Here's how the part is built. I have some questions about the finished solid (model axes, mm). Give positions to 0.01 mm unless a question says otherwise; leave off trailing zeros.
Q1. Suppose I cut it at A-A (z = 1.3). Count the separate pieces of the cut face and the enclosed holes in it, and give its area (3 significant figures).
Q2. I need wall thicknesses on probe 1 along Y at (x, z) = (66.04, 1.15) (1 decimal); probe 2 along X at (y, z) = (-14, 1.35); probe 3 along Y at (x, z) = (-20.32, 0.6) (1 decimal). Which ranges of each line are inside material? Lowest first, please.
Q3. I'm going to push flat-ended pins straight in: P1, Ø1.5, axis at x = 37.5, y = 124, coming from the -Z side; P2, Ø0.8, axis at y = -15.5, z = 0.5, coming from the +X side; P3, Ø0.8, axis at x = 59.5, z = 0.5, coming from the +Y side. Where does each tip first touch, or does it pass through?
```python
from build123d import *

# Parameters (mm, degrees)
F0_W     = 1.5875
F0_H     = 10
F0_H_2   = 20
F0_W_2   = 1.74625
F0_H_3   = 5.15
F0_W_3   = 5.15
F0_H_4   = 1.74625
F0_W_4   = 200
F0_H_5   = 1.5875
F0_W_5   = 50
F0_R     = 1.4732
F0_W_6   = 25
F0_H_6   = 30
F0_W_7   = 10
F0_W_8   = 20
F1_DEPTH = 1.5875


# Not quite as in the source:
# - a length typed as a fraction of an inch, garbled in the dataset ("3 / 203.2 mm" for 3/8 in), is restored


with BuildPart() as f1:
    # F0 (on Top) → F1 (new body)
    with BuildSketch(Plane.XY):
        with Locations((-100.79375, 176.5875)):
            Rectangle(F0_W, F0_H)
        with Locations((-100.79375, 36.5875)):
            Rectangle(F0_W, F0_H)
        with Locations((-100.79375, 61.5875)):
            Rectangle(F0_W, F0_H_2)
        with Locations((100.79375, 176.5875)):
            Rectangle(F0_W, F0_H)
        with Locations((100.79375, 36.5875)):
            Rectangle(F0_W, F0_H)
        with Locations((100.79375, 61.5875)):
            Rectangle(F0_W, F0_H_2)
        Polygon((100, 10), (100, 20), (-100, 20), (-100, 10), (-100, -10), (-100, -20), (100, -20), (100, -10), align=None)
        with Locations((-64.2875, -15)):
            Rectangle(F0_W_2, F0_H_3, mode=Mode.SUBTRACT)
        with Locations((-58.414375, -15)):
            Rectangle(F0_W_3, F0_H_4, mode=Mode.SUBTRACT)
        with Locations((-64.2875, 15)):
            Rectangle(F0_W_2, F0_H_3, mode=Mode.SUBTRACT)
        with Locations((-58.414375, 15)):
            Rectangle(F0_W_3, F0_H_4, mode=Mode.SUBTRACT)
        with Locations((-38.414375, -15)):
            Rectangle(F0_W_3, F0_H_4, mode=Mode.SUBTRACT)
        with Locations((-14.2875, -15)):
            Rectangle(F0_W_2, F0_H_3, mode=Mode.SUBTRACT)
        with Locations((-38.414375, 15)):
            Rectangle(F0_W_3, F0_H_4, mode=Mode.SUBTRACT)
        with Locations((-14.2875, 15)):
            Rectangle(F0_W_2, F0_H_3, mode=Mode.SUBTRACT)
        with Locations((14.2875, -15)):
            Rectangle(F0_W_2, F0_H_3, mode=Mode.SUBTRACT)
        with Locations((38.414375, -15)):
            Rectangle(F0_W_3, F0_H_4, mode=Mode.SUBTRACT)
        with Locations((14.2875, 15)):
            Rectangle(F0_W_2, F0_H_3, mode=Mode.SUBTRACT)
        with Locations((38.414375, 15)):
            Rectangle(F0_W_3, F0_H_4, mode=Mode.SUBTRACT)
        with Locations((58.414375, -15)):
            Rectangle(F0_W_3, F0_H_4, mode=Mode.SUBTRACT)
        with Locations((64.2875, -15)):
            Rectangle(F0_W_2, F0_H_3, mode=Mode.SUBTRACT)
        with Locations((58.414375, 15)):
            Rectangle(F0_W_3, F0_H_4, mode=Mode.SUBTRACT)
        with Locations((64.2875, 15)):
            Rectangle(F0_W_2, F0_H_3, mode=Mode.SUBTRACT)
        Polygon((-100, 20), (100, 20), (100, 30), (75, 30), (25, 30), (-25, 30), (-75, 30), (-100, 30), align=None)
        with Locations((0, -25)):
            Rectangle(F0_W_4, F0_H)
        with Locations((-100.79375, 0)):
            Rectangle(F0_W, F0_H_2)
        with Locations((100.79375, 0)):
            Rectangle(F0_W, F0_H_2)
        with Locations((100.79375, 25)):
            Rectangle(F0_W, F0_H)
        with Locations((100.79375, -25)):
            Rectangle(F0_W, F0_H)
        with Locations((-100.79375, 25)):
            Rectangle(F0_W, F0_H)
        with Locations((-100.79375, -25)):
            Rectangle(F0_W, F0_H)
        Polygon((101.5875, -30), (100, -30), (-100, -30), (-100, -31.5875), (101.5875, -31.5875), align=None)
        with Locations((-100.79375, 30.79375)):
            Rectangle(F0_W, F0_H_5)
        with Locations((0, 30.79375)):
            Rectangle(F0_W_5, F0_H_5)
        with Locations((100.79375, 30.79375)):
            Rectangle(F0_W, F0_H_5)
        with Locations((-100.79375, -30.79375)):
            Rectangle(F0_W, F0_H_5)
        Polygon((75, 31.5875), (100, 31.5875), (100, 41.5875), (100, 51.5875), (100, 71.5875), (100, 91.5875), (100, 121.5875), (100, 141.5875), (100, 161.5875), (100, 171.5875), (100, 181.5875), (90, 181.5875), (80, 181.5875), (60, 181.5875), (40, 181.5875), (20, 181.5875), (-20, 181.5875), (-40, 181.5875), (-60, 181.5875), (-80, 181.5875), (-90, 181.5875), (-100, 181.5875), (-100, 171.5875), (-100, 161.5875), (-100, 141.5875), (-100, 121.5875), (-100, 91.5875), (-100, 71.5875), (-100, 51.5875), (-100, 41.5875), (-100, 31.5875), (-75, 31.5875), (-25, 31.5875), (25, 31.5875), align=None)
        with Locations((-66.04, 68.5975)):
            Circle(F0_R, mode=Mode.SUBTRACT)
        with Locations((-20.32, 37.8975)):
            Circle(F0_R, mode=Mode.SUBTRACT)
        with Locations((-20.32, 58.2175)):
            Circle(F0_R, mode=Mode.SUBTRACT)
        with Locations((20.32, 37.8975)):
            Circle(F0_R, mode=Mode.SUBTRACT)
        with Locations((20.32, 58.2175)):
            Circle(F0_R, mode=Mode.SUBTRACT)
        with Locations((66.04, 68.5975)):
            Circle(F0_R, mode=Mode.SUBTRACT)
        with Locations((-66.04, 175.2775)):
            Circle(F0_R, mode=Mode.SUBTRACT)
        with Locations((66.04, 175.2775)):
            Circle(F0_R, mode=Mode.SUBTRACT)
        with Locations((87.5, 30.79375)):
            Rectangle(F0_W_6, F0_H_5)
        with Locations((-87.5, 30.79375)):
            Rectangle(F0_W_6, F0_H_5)
        with Locations((-100.79375, 106.5875)):
            Rectangle(F0_W, F0_H_6)
        with Locations((-100.79375, 151.5875)):
            Rectangle(F0_W, F0_H_2)
        with Locations((100.79375, 151.5875)):
            Rectangle(F0_W, F0_H_2)
        with Locations((100.79375, 106.5875)):
            Rectangle(F0_W, F0_H_6)
        with Locations((95, 182.38125)):
            Rectangle(F0_W_7, F0_H_5)
        with Locations((100.79375, 182.38125)):
            Rectangle(F0_W, F0_H_5)
        with Locations((-100.79375, 182.38125)):
            Rectangle(F0_W, F0_H_5)
        with Locations((-95, 182.38125)):
            Rectangle(F0_W_7, F0_H_5)
        with Locations((-70, 182.38125)):
            Rectangle(F0_W_8, F0_H_5)
        with Locations((-30, 182.38125)):
            Rectangle(F0_W_8, F0_H_5)
        with Locations((70, 182.38125)):
            Rectangle(F0_W_8, F0_H_5)
        with Locations((30, 182.38125)):
            Rectangle(F0_W_8, F0_H_5)
    extrude(amount=F1_DEPTH)


solid = f1.part
```
Solutions:
1. separate pieces: 1
1. enclosed holes: 26
1. area: 42,900 mm2
2. probe 1: y = -31.6 to 30, 31.6 to 67.1, 70.1 to 173.8, 176.8 to 183.2
2. probe 2: x = -100 to -65.16, -63.41 to -15.16, -13.41 to 13.41, 15.16 to 63.41, 65.16 to 100
2. probe 3: y = -31.6 to 36.4, 39.4 to 56.7, 59.7 to 183.2
3. P1: stops at z = 0
3. P2: stops at x = 100
3. P3: stops at y = 181.59
